CAD build for the part. Positions are in the model's coordinates, mm. Round coordinates to 2 decimals unless told otherwise and drop trailing zeros. Order: outer loops, then holes, each group sorted by start corner. A loop starts at its lowest first (then second) coordinate and runs counter-clockwise, first axis right, second up. Notation, with made-up numbers: (58, 3.5) - (82, 3.5) arc R27 cw to (82, 31.5) - close; hole circle Ø1 at (-9, -30). An arc over 180 degrees is marked (long way). Write item = value, one per line.
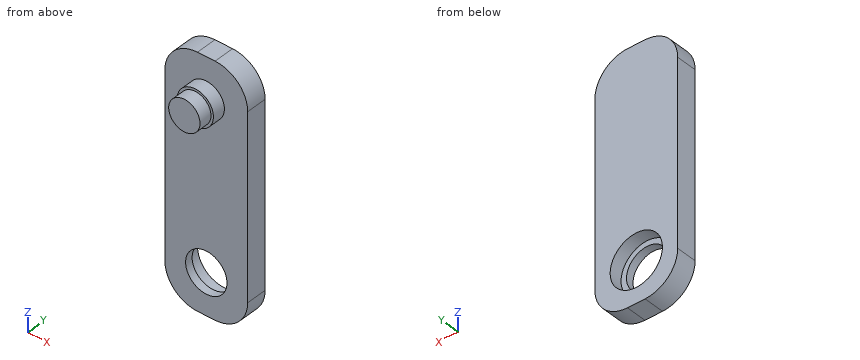
from build123d import *

# Parameters (mm, degrees)
SKETCH1_W           = 25.4
SKETCH1_H           = 76.2
BOSS_EXTRUDE1_DEPTH = 6.35
SKETCH5_R           = 8.016875
CUT_EXTRUDE1_DEPTH  = 3.96875
SKETCH6_R           = 6.35
CUT_EXTRUDE2_DEPTH  = 81.419841933
BOSS_EXTRUDE2_START = -6.35
SKETCH7_R           = 5.55625
BOSS_EXTRUDE2_DEPTH = 4
SKETCH8_R           = 4.805
BOSS_EXTRUDE3_DEPTH = 4
FILLET1_R           = 10


with BuildPart() as part:
    # Sketch1 → Boss-Extrude1 (new body)
    with BuildSketch(Plane(origin=(0, 0, 0), x_dir=(1, 0, 0), z_dir=(0, 1, 0))):
        with Locations((12.7, 38.1)):
            Rectangle(SKETCH1_W, SKETCH1_H)
    extrude(amount=BOSS_EXTRUDE1_DEPTH)

    # Sketch5 → Cut-Extrude1 (cut)
    with BuildSketch(Plane(origin=(0, 6.35, 0), x_dir=(1, 0, 0), z_dir=(0, 1, 0))):
        with Locations(Location((12.7, 63.5, 0), (0, 0, 270))):
            Circle(SKETCH5_R)
    extrude(amount=-CUT_EXTRUDE1_DEPTH, mode=Mode.SUBTRACT)

    # Sketch6 → Cut-Extrude2 (cut, through all)
    with BuildSketch(Plane(origin=(0, 2.38125, 0), x_dir=(1, 0, 0), z_dir=(0, 1, 0))):
        with Locations(Location((12.7, 63.5, 0), (0, 0, 270))):
            Circle(SKETCH6_R)
    extrude(amount=-CUT_EXTRUDE2_DEPTH, mode=Mode.SUBTRACT)

    # Sketch7 → Boss-Extrude2 (add)
    with BuildSketch(Plane(origin=(0, 6.35, 0), x_dir=(1, 0, 0), z_dir=(0, 1, 0)).offset(BOSS_EXTRUDE2_START)):
        with Locations(Location((12.7, 12.7, 0), (0, 0, 90))):
            Circle(SKETCH7_R)
    extrude(amount=-BOSS_EXTRUDE2_DEPTH)

    # Sketch8 → Boss-Extrude3 (add)
    with BuildSketch(Plane.XZ.offset(4)):
        with Locations(Location((12.7, -12.7, 0), (0, 0, 270))):
            Circle(SKETCH8_R)
    extrude(amount=BOSS_EXTRUDE3_DEPTH)

    # Fillet1
    fillet1_edges = [part.edges().sort_by_distance(p)[0] for p in [
        (0, 3.175, -76.2),
        (25.4, 3.175, -76.2),
        (25.4, 3.175, 0),
        (0, 3.175, 0),
    ]]
    fillet(fillet1_edges, radius=FILLET1_R)


solid = part.part
(1) Band-saw the part on A-A on z = -63.5. List the corners of the cut face in (x, y), plus the area to 3 significant figures.
Solved:
outline = (0, 0) - (6.35, 0) - (6.35, 2.38) - (4.68, 2.38) - (4.68, 6.35) - (0, 6.35) - close; (19.05, 0) - (25.4, 0) - (25.4, 6.35) - (20.72, 6.35) - (20.72, 2.38) - (19.05, 2.38) - close
area = 67.4 mm²
(2) Probe line 1 along X through (y, z) = (1.65, -63.5); line 2 along X through (y, z) = (4.1, -63.5); line 3 along Y through (x, z) = (17, -69.5). List the from-to ranges inside material, lowest first.
Solved:
line_1 = 0 to 6.35, 19.05 to 25.4
line_2 = 0 to 4.68, 20.72 to 25.4
line_3 = 0 to 2.38
(3) Drop flat-ended pins along their axis: pin 1 (8 mm diameter, centred on x = 17, z = -57, fed in from -Y); pin 2 (13 mm diameter, centred on x = 11, z = -62, fed in from +Y); pin 3 (2 mm diameter, centred on x = 12.5, y = -1.5, fed in from +Z). Give the stop position or say it passes through.
Solved:
pin_1 = 0
pin_2 = 6.35
pin_3 = -7.14
(4) Band-saw the part on B-B on x = 12.7. List the corners of the cut face in (y, z) (3 decimals), plus the area to 3 significant figures.
Solved:
outline = (-8, -17.505) - (-4, -17.505) - (-4, -18.256) - (0, -18.256) - (0, -57.15) - (2.381, -57.15) - (2.381, -55.483) - (6.35, -55.483) - (6.35, 0) - (0, 0) - (0, -7.144) - (-4, -7.144) - (-4, -7.895) - (-8, -7.895) - close; (0, -76.2) - (6.35, -76.2) - (6.35, -71.517) - (2.381, -71.517) - (2.381, -69.85) - (0, -69.85) - close
area = 473 mm²
(5) Band-saw the part on C-C on z = -12.7. List the corners of the cut face in (x, y) (3 decimals).
Solved:
outline = (0, 0) - (7.144, 0) - (7.144, -4) - (7.895, -4) - (7.895, -8) - (17.505, -8) - (17.505, -4) - (18.256, -4) - (18.256, 0) - (25.4, 0) - (25.4, 6.35) - (0, 6.35) - close
(6) Band-saw the part on D-D on y = -5.5. List the corners of the cut face in (x, z) (3 decimals).
Solved:
outline = circle Ø9.61 at (12.7, -12.7)
